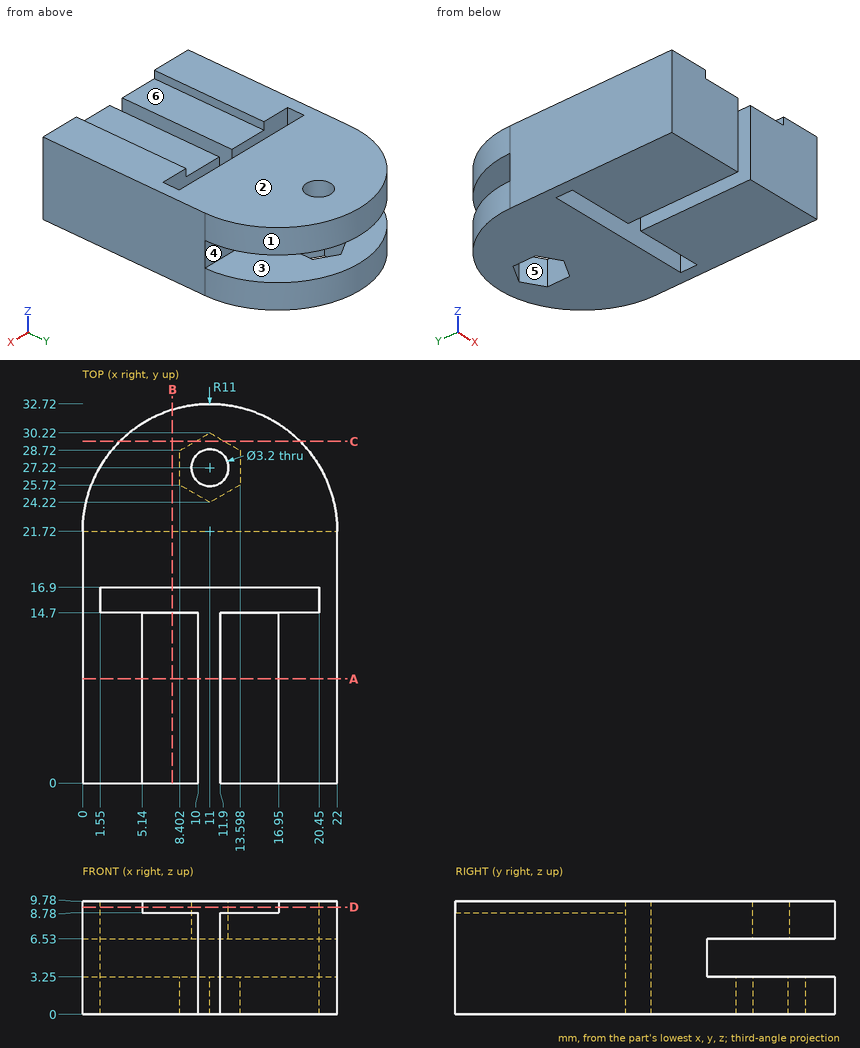
Input: dimensioned drawing with shaded views. Units: mm. Origin: part minimum x, y, z. A direction names the side the tool comes from. Coordinates: 2 decimals unless noted, no trailing zeros. Write each loop counter-clockwise with the first axis right and the second up, starting at its lowest first coordinate (ties: lowest second). Pieces come first, ordered by that corner, then holes. Notation, with made-up numbers: M 33.25,-12 L 59.25,-12 A12 cw 59.25,0 Z; hole C -1.75,-12.5 d2. An arc over 180 degrees is marked long. Answer as CSV lines item,"result". Start each with the question number.
Q1. Cut plane D-D on z = 9.25. Return the cut outline in (x, y).
Q2. Line query: line 1 (Y direction, x = 11, z = 7.3); line 2 (X direction, y = 4.5, z = 4.75); line 3 (Z direction, x = 20, y = 27). Output: solid intervals per line, ascending. Write a range as from..to.
Q3. Cut plane B-B on x = 7.75. Return the cut outline in (y, z), then the cut area to 4 significant figures.
Q4. Pin query (flat end, axial travel): P1, Ø5.5, axis at x = 7.5, y = 28.5, coming from the -Z side; P2, Ø3.5, axis at y = 27.5, z = 1.5, coming from the +X side (3 decimals); P3, Ø8, axis at x = 10, y = 10, coming from the +Z side; P4, Ø2, axis at x = 13.5, z = 8, coming from the +Y side. Return the tip coordinate at first contact, or that it passes through.
Q5. Cut plane C-C on y = 29.5. Return the cut outline in (x, z).
Q6. Reachability of the marked faces 4, 5 and 6 from +Z, -Z, +X, -X, +Y, -Y: full face, straight path, thin tool, end or side. Return the list, or none.
Q7. Cut plane A-A on y = 9. Return the cut outline in (x, z), then the cut area to 3 significant figures.
Q8. Mould query, pull axis Z, two halves, no side actions, for the marked faces 1, 2 and 3. Classes: released by +Z, released by -Z, zero draft, split by the parting line, or undercut.
Findings below:
1,outline,"M 0,0 L 5.14,0 L 5.14,14.7 L 1.55,14.7 L 1.55,16.9 L 20.45,16.9 L 20.45,14.7 L 16.95,14.7 L 16.95,0 L 22,0 L 22,21.72 A11 ccw 0,21.72 Z; hole C 11,27.22 d3.2"
2,line 1,"y = 16.9..25.62, 28.82..32.72"
2,line 2,"x = 0..10, 11.9..22"
2,line 3,"z = 0..3.25, 6.53..9.78"
3,outline,"M 0,0 L 14.7,0 L 14.7,8.78 L 0,8.78 Z; M 16.9,0 L 32.23,0 L 32.23,3.25 L 21.72,3.25 L 21.72,6.53 L 32.23,6.53 L 32.23,9.78 L 16.9,9.78 Z"
3,area,"244.5 mm2"
4,P1,"stops at z = 0"
4,P2,"stops at x = 21.235"
4,P3,"stops at z = 8.78"
4,P4,"stops at y = 32.62"
5,outline,"M 3.22,0 L 9.75,0 L 9.75,3.25 L 3.22,3.25 Z; M 3.22,6.53 L 18.78,6.53 L 18.78,9.78 L 3.22,9.78 Z; M 12.25,0 L 18.78,0 L 18.78,3.25 L 12.25,3.25 Z"
6,face 4,"+X, -X, +Y"
6,face 5,"-Z"
6,face 6,"+Z, -Y"
7,outline,"M 0,0 L 10,0 L 10,8.78 L 5.14,8.78 L 5.14,9.78 L 0,9.78 Z; M 11.9,0 L 22,0 L 22,9.78 L 16.95,9.78 L 16.95,8.78 L 11.9,8.78 Z"
7,area,"187 mm2"
8,face 1,"zero draft"
8,face 2,"released by +Z"
8,face 3,"undercut"
